Job drawing, mm, ordinate dimensions from the low corner. One solid piece. A direction names the side the tool comes from. Give positions to 0.01 mm unless a question says otherwise; leave off trailing zeros. Order: outer loops, then holes, each group sorted by start corner. A loop starts at its lowest first (then second) coordinate and runs counter-clockwise, first axis right, second up. Notation, with made-up numbers: (37.25, 55) -> (58.25, 55) arc R26 ccw to (58.25, 71) -> close; hole circle Ø10 at (-5, 9.5). An arc over 180 degrees is marked (long way). Use CSV: the item, a comma, the result in double quotes. Start each with the question number.
1. Cut at A-A on x = 52. List the corners of the cut face in (y, z) (3 decimals), then the cut area to 3 significant figures.
2. Cut at D-D on y = 31. List the corners of the cut face in (x, z), then the cut area to 3 significant figures.
3. Cut at B-B on z = 17.25. List the corners of the cut face in (x, y), then the cut area to 3 significant figures.
4. Cut at C-C on x = 44. List the corners of the cut face in (y, z), then the cut area to 3 significant figures.
5. Wall check: line 1 (Y direction, x = 41.5, z = 19.25); line 2 (X direction, y = 55, z = 6.5); line 3 (Z direction, x = 34.5, y = 25.5). Give the ranges that are in metal, low to high. Write a range as from..to.
6. 3-axis set-ups, long thin cutter, end or side, ignore diameter. For the marked faces 5 and 6: which of +Z, -Z, +X, -X, +Y, -Y reach the whole face in a straight line?
7. Pull direction Y, two halves, no side cores. Call the marked faces 1, 2, 3 and 4: released by +Y, released by -Y, zero draft, split by the parting line, or undercut.
8. Drop a flat-ended pin along its axis: pin 1 (2 mm diameter, centred on x = 15, y = 15.5, fed in from +Z). Give the stop position or say it passes through.
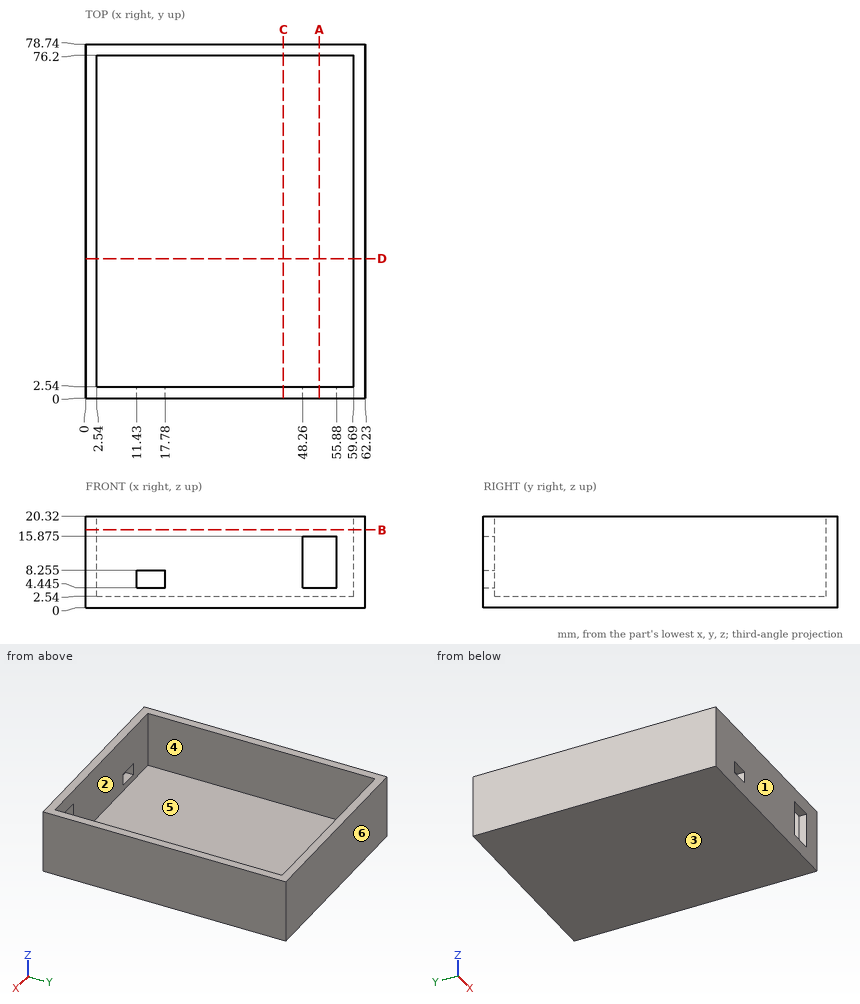
Verdict:
1,outline,"(0, 0) -> (78.74, 0) -> (78.74, 20.32) -> (76.2, 20.32) -> (76.2, 2.54) -> (2.54, 2.54) -> (2.54, 4.445) -> (0, 4.445) -> close; (0, 15.875) -> (2.54, 15.875) -> (2.54, 20.32) -> (0, 20.32) -> close"
1,area,"261 mm^2"
2,outline,"(0, 0) -> (62.23, 0) -> (62.23, 20.32) -> (59.69, 20.32) -> (59.69, 2.54) -> (2.54, 2.54) -> (2.54, 20.32) -> (0, 20.32) -> close"
2,area,"248 mm^2"
3,outline,"(0, 0) -> (62.23, 0) -> (62.23, 78.74) -> (0, 78.74) -> close; hole (2.54, 2.54) -> (59.69, 2.54) -> (59.69, 76.2) -> (2.54, 76.2) -> close"
3,area,"690 mm^2"
4,outline,"(0, 0) -> (78.74, 0) -> (78.74, 20.32) -> (76.2, 20.32) -> (76.2, 2.54) -> (2.54, 2.54) -> (2.54, 20.32) -> (0, 20.32) -> close"
4,area,"290 mm^2"
5,line 1,"0..2.54, 76.2..78.74"
5,line 2,"0..2.54, 59.69..62.23"
5,line 3,"0..2.54"
6,face 5,"+Z"
6,face 6,"+Z, -Z, +X, -X, +Y"
7,face 1,"released by -Y"
7,face 2,"undercut"
7,face 3,"zero draft"
7,face 4,"undercut"
8,pin 1,"z = 2.54"
